Source: CAD feature listing. Evaluate the final solid. Frame: model axes, mm. A direction names the side the tool comes from. Give positions to 0.01 mm unless a question says otherwise; leave off trailing zeros. Write each loop counter-clockwise with the first axis right and the second up, starting at its lowest first coordinate (ties: lowest second). Pieces come first, ordered by that corner, then holes. Notation, with made-up numbers: M 71.5,65.5 L 101.5,65.5 A19 cw 101.5,101.5 Z; hole C -16.75,75.5 d7. An arc over 180 degrees is marked long. Use CSV: the item, a comma, the result in double quotes. Start each with the question number.
from build123d import *

# Parameters (mm, degrees)
F0_R     = 3.175
F0_R_2   = 2.878099
F1_DEPTH = 3.175
F3_ANGLE = 41


with BuildPart() as f1:
    # F0 (on Right) → F1 (new body)
    with BuildSketch(Plane.YZ):
        with BuildLine():
            Line((-0.683293, -22.206229), (-21.279692, -6.062372))
            ThreePointArc((-21.279692, -6.062372), (-31.89988, -6.809987), (-32.223099, -17.45155))
            Line((-32.223099, -17.45155), (-32.127586, -17.5618))
            Line((-32.127586, -17.5618), (-3.144408, -51.016742))
            ThreePointArc((-3.144408, -51.016742), (4.260096, -54.808331), (12.221904, -52.397431))
            Line((12.221904, -52.397431), (59.870195, -14.049133))
            Line((59.870195, -14.049133), (63.249417, -11.329467))
            ThreePointArc((63.249417, -11.329467), (62.611086, 11.0927), (40.187851, 10.493082))
            ThreePointArc((40.187851, 10.493082), (40.178419, 10.48314), (40.168995, 10.47319))
            Line((40.168995, 10.47319), (10.036033, -21.370629))
            ThreePointArc((10.036033, -21.370629), (4.839042, -23.875239), (-0.683293, -22.206229))
        make_face()
        with Locations((5.254567, -43.740418)):
            Circle(F0_R, mode=Mode.SUBTRACT)
        with Locations((18.772386, -30.935138)):
            Circle(F0_R_2, mode=Mode.SUBTRACT)
        with Locations((-26.176328, -12.30952)):
            Circle(F0_R, mode=Mode.SUBTRACT)
        with Locations((51.699796, -0.4381)):
            Circle(F0_R, mode=Mode.SUBTRACT)
    extrude(amount=F1_DEPTH)


with BuildPart() as f1_1:
    # F3: moved
    add(f1.part.rotate(Axis((-5.653633, 0, 21.454556), (-1, 0, 0)), F3_ANGLE))


solid = f1_1.part
Item 1: Contact query for flat-ended pins moving along their axis: pin 1 Ø6 at (y, z) = (-27, 2) entering from +X; pin 2 Ø1 at (x, z) = (0.5, -38) entering from -Y; pin 3 Ø1.5 at (x, y) = (1.5, 13) entering from -Z. Output: stop coordinate, or through.
Item 2: Pull-direction query (Z, two-part tool) for faces 3 (the cylindrical face through (1.565, 22.353, -26.8)), 4 (the cylindrical face through (1.57, -26.02, -15.98)), 5 (the cylindrical face through (1.565, 40.485, -27.79)); classes: released by +Z, released by -Z, zero draft, split by the parting line, or undercut.
Item 3: Set-up query: faces 1 (the flat face through (1.57, 1.6, -15.29)), 2 (the flat face through (3.175, -6, -27)). Return all of +Z, -Z, +X, -X, +Y, -Y with unobstructed straight access to the full face (end or side cutting, diameter ignored); none if empty.
Item 4: Material intervals for probe 1 along Y at (x, z) = (1.4, -28.5); probe 2 along Z at (x, y) = (1, -40); probe 3 along Y at (x, z) = (0.75, -11), sorted ascending.
Item 5: Section B-B (y = 11.5). Return the cut outline in (x, z) (3 decimals), plus the area to 3 significant figures.
Item 6: Section A-A (x = 0.9). State how many separate pieces and enclosed holes the cut face has, plus the area to 3 significant figures.
Item 7: Section C-C (z = -7). Return the cut outline in (x, y) (3 decimals).
Output values:
1,pin 1,"passes through"
1,pin 2,"stops at y = -47.96"
1,pin 3,"stops at z = -44.31"
2,face 3,"undercut"
2,face 4,"released by +Z"
2,face 5,"split by the parting line"
3,face 1,"+Z, +X, -X"
3,face 2,"+Z, -Z, +X, +Y, -Y"
4,probe 1,"y = -49.91 to -40.48, -37.13 to -22.36, -18.04 to 21.52, 27.79 to 40.52"
4,probe 2,"z = -42.24 to -34.14, -28.25 to 10.61, 15.68 to 20.85"
4,probe 3,"y = -49.88 to -29.17"
5,outline,"M 0,-44.225 L 3.175,-44.225 L 3.175,-14.321 L 0,-14.321 Z"
5,area,"94.9 mm2"
6,separate pieces,"1"
6,enclosed holes,"4"
6,area,"2,970 mm2"
7,outline,"M 0,-49.878 L 3.175,-49.878 L 3.175,-29.94 L 0,-29.94 Z"
